The listing builds one solid part. Answer for the finished solid, in the listing's coordinates (mm). A direction names the side the tool comes from. Coordinates: 2 decimals unless noted, no trailing zeros. Order: outer loops, then holes, each group sorted by start corner. A loop starts at its lowest first (then second) coordinate and runs counter-clockwise, first axis right, second up.
from build123d import *

# Parameters (mm, degrees)
SKETCH1_R           = 2.265
BOSS_EXTRUDE1_DEPTH = 3
CUT_EXTRUDE1_DEPTH  = 3
SKETCH3_W           = 6.5
SKETCH3_H           = 20
CUT_EXTRUDE2_DEPTH  = 3
BOSS_EXTRUDE2_DEPTH = 3
SKETCH5_W           = 6.5
SKETCH5_H           = 20
BOSS_EXTRUDE3_DEPTH = 3
FILLET1_R           = 0.6


with BuildPart() as part:
    # Sketch1 → Boss-Extrude1 (new body)
    with BuildSketch(Plane(origin=(0, 0, 0), x_dir=(1, 0, 0), z_dir=(0, 1, 0))):
        with BuildLine():
            Line((4.265, 0), (87.735, 0))
            ThreePointArc((87.735, 0), (95.015810422, 3.015810422), (92, -4.265))
            Line((92, -4.265), (92, -58.735))
            ThreePointArc((92, -58.735), (95.015810422, -66.015810422), (87.735, -63))
            Line((87.735, -63), (4.265, -63))
            ThreePointArc((4.265, -63), (-3.015810422, -66.015810422), (0, -58.735))
            Line((0, -58.735), (0, -4.265))
            ThreePointArc((0, -4.265), (-3.015810422, 3.015810422), (4.265, 0))
        make_face()
        with Locations(Location((0, 0, 0), (0, 0, 270))):
            Circle(SKETCH1_R, mode=Mode.SUBTRACT)
        with Locations(Location((92, 0, 0), (0, 0, 270))):
            Circle(SKETCH1_R, mode=Mode.SUBTRACT)
        with Locations(Location((92, -63, 0), (0, 0, 270))):
            Circle(SKETCH1_R, mode=Mode.SUBTRACT)
        with Locations(Location((0, -63, 0), (0, 0, 270))):
            Circle(SKETCH1_R, mode=Mode.SUBTRACT)
    extrude(amount=BOSS_EXTRUDE1_DEPTH)

    # Sketch2 → Cut-Extrude1 (cut)
    with BuildSketch(Plane(origin=(0, 3, 0), x_dir=(1, 0, 0), z_dir=(0, 1, 0))):
        Polygon((6.5, -4), (66.5, -4), (66.5, -14), (66.5, -18), (58.5, -18), (58.5, -14), (6.5, -14), align=None)
    extrude(amount=-CUT_EXTRUDE1_DEPTH, mode=Mode.SUBTRACT)

    # Sketch3 → Cut-Extrude2 (cut)
    with BuildSketch(Plane(origin=(0, 3, 0), x_dir=(1, 0, 0), z_dir=(0, 1, 0))):
        with Locations((3.25, -31.5)):
            Rectangle(SKETCH3_W, SKETCH3_H)
    extrude(amount=-CUT_EXTRUDE2_DEPTH, mode=Mode.SUBTRACT)

    # Sketch4 → Boss-Extrude2 (add)
    with BuildSketch(Plane(origin=(0, 3, 0), x_dir=(1, 0, 0), z_dir=(0, 1, 0))):
        with BuildLine():
            Line((-2.7, -15.5), (0, -14.9))
            Line((0, -14.9), (0, -21.5))
            Line((0, -21.5), (-2.5, -21.5))
            ThreePointArc((-2.5, -21.5), (-2.853553391, -21.353553391), (-3, -21))
            Line((-3, -21), (-3, -15.8))
            ThreePointArc((-3, -15.8), (-2.912132034, -15.587867966), (-2.7, -15.5))
        make_face()
        with BuildLine():
            Line((-3, -42), (-3, -47.2))
            ThreePointArc((-3, -47.2), (-2.912132034, -47.412132034), (-2.7, -47.5))
            Line((-2.7, -47.5), (0, -48.1))
            Line((0, -48.1), (0, -41.5))
            Line((0, -41.5), (-2.5, -41.5))
            ThreePointArc((-2.5, -41.5), (-2.853553391, -41.646446609), (-3, -42))
        make_face()
    extrude(amount=-BOSS_EXTRUDE2_DEPTH)

    # Sketch5 → Boss-Extrude3 (add)
    with BuildSketch(Plane(origin=(0, 3, 0), x_dir=(1, 0, 0), z_dir=(0, 1, 0))):
        with Locations((3.25, -31.5)):
            Rectangle(SKETCH5_W, SKETCH5_H)
    extrude(amount=-BOSS_EXTRUDE3_DEPTH)

    # Fillet1
    fillet1_edges = [part.edges().sort_by_distance(p)[0] for p in [
        (0, 1.5, 48.1),
        (0, 1.5, 41.5),
        (0, 1.5, 21.5),
        (92, 1.5, 4.265),
        (92, 1.5, 58.735),
        (87.735, 1.5, 63),
        (4.265, 1.5, 63),
        (0, 1.5, 58.735),
        (0, 1.5, 4.265),
        (4.265, 1.5, 0),
        (87.735, 1.5, 0),
        (0, 1.5, 14.9),
    ]]
    fillet(fillet1_edges, radius=FILLET1_R)


solid = part.part
(1) Find section D-D on x = 83.5. Determine the outline of the cut face in (y, z).
(2) Find the intervals of material crossed by probe 1 along Z at (x, y) = (66, 1.15); probe 2 along X at (y, z) = (0.75, 11); probe 3 along Z at (x, y) = (12, 0.2), in increasing order.
(3) The mould has two halves that part along Z. Classify faces 3 (the flat face through (45, 0, 39)), 4 (the flat face through (45, 1, 0)), 5 (the flat face through (0, 2, 32)): pulls with the +Z half, pulls with the -Z half, needs draft (parallel to the pull), parting line crosses it, or undercut.
(4) Find section B-B on z = 39. Determine the outline of the cut face in (x, y), then the cut area to 3 significant figures.
(5) Find section C-C on y = 1.6. Count the separate pieces of the cut face and the enclosed holes in it, then the cut area to 3 significant figures.
(6) A tool of negligible diameter and unlimited length cuts with its end or side. For faces 1 (the flat face through (0, 1, 53)), 2 (the flat face through (58.5, 2, 16)), from which of +Z, -Z, +X, -X, +Y, -Y can it reach the whole face along a straight path? Write none if from no direction.
(7) Given pin 1 Ø0.9 at (y, z) = (1.5, 13) entering from -X; pin 2 Ø7 at (x, z) = (92, 0) entering from -Y; pin 3 Ø1 at (x, y) = (-1.5, 2) entering from -Z; pin 4 Ø1 at (x, y) = (-1.5, 2) entering from +Z, each flat-ended and moving along its own axis, determine where each tip first touches the part or whether it passes through.
(8) Find section A-A on x = 10. Determine the outline of the cut face in (y, z).
Resolved:
1. outline: (0, 0) - (3, 0) - (3, 63) - (0, 63) - close
2. probe 1: z = 0 to 4, 18 to 63
2. probe 2: x = 0 to 6.5, 66.5 to 92
2. probe 3: z = 0 to 4, 14 to 63
3. face 3: needs draft
3. face 4: pulls with the -Z half
3. face 5: undercut
4. outline: (0, 0) - (92, 0) - (92, 3) - (0, 3) - close
4. area: 276 mm2
5. separate pieces: 1
5. enclosed holes: 5
5. area: 5,310 mm2
6. face 1: -X, +Y, -Y
6. face 2: +Y, -Y
7. pin 1: stops at x = 0
7. pin 2: stops at y = 0
7. pin 3: stops at z = -4.15
7. pin 4: stops at z = 67.15
8. outline: (0, 0) - (3, 0) - (3, 4) - (0, 4) - close; (0, 14) - (3, 14) - (3, 63) - (0, 63) - close
